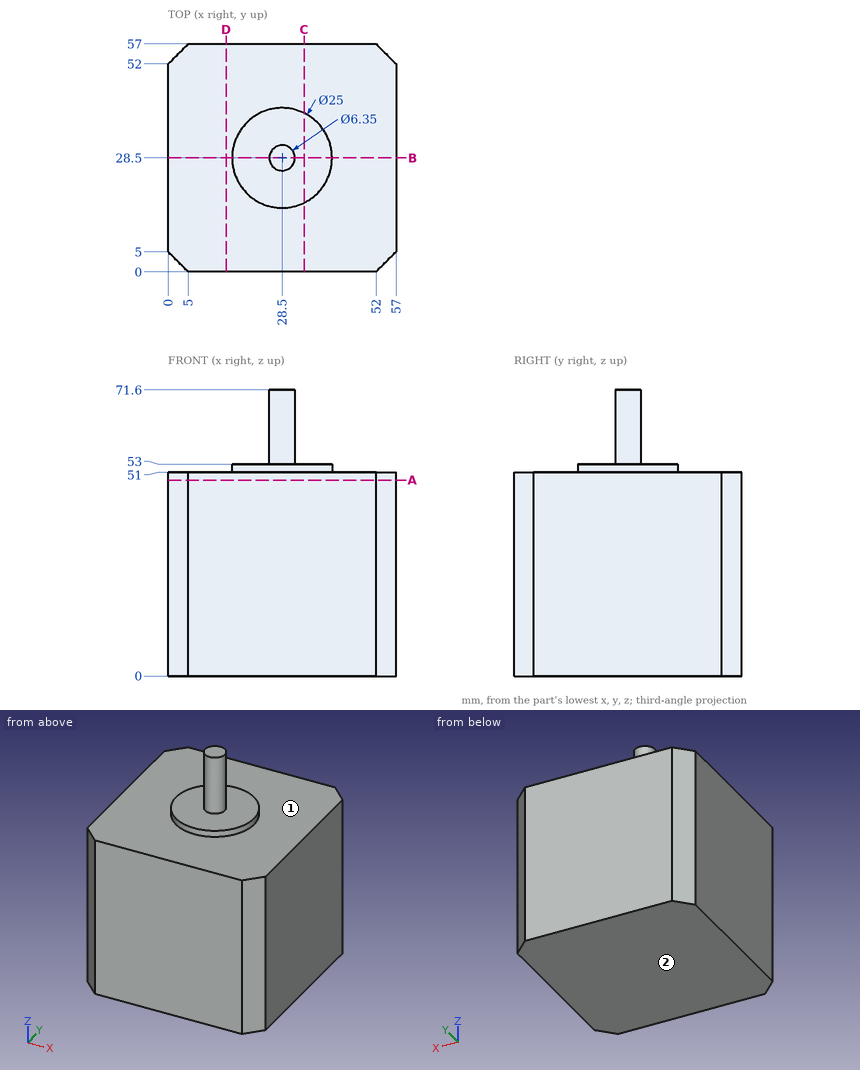
Input: dimensioned drawing with shaded views. Units: mm. Origin: part minimum x, y, z. A direction names the side the tool comes from. Coordinates: 2 decimals unless noted, no trailing zeros. Order: outer loops, then holes, each group sorted by start corner. A loop starts at its lowest first (then second) coordinate and runs counter-clockwise, first axis right, second up.
Item 1: Section query A-A (z = 49). Output: boundary loops of the cut face in (x, y), then the cut area to 3 significant figures.
Answer:
outline: (0, 5) - (5, 0) - (52, 0) - (57, 5) - (57, 52) - (52, 57) - (5, 57) - (0, 52) - close
area: 3,200 mm2
Item 2: Section query C-C (x = 34). Output: boundary loops of the cut face in (y, z).
Answer:
outline: (0, 0) - (57, 0) - (57, 51) - (39.72, 51) - (39.72, 53) - (17.28, 53) - (17.28, 51) - (0, 51) - close
Item 3: Section query B-B (y = 28.5). Output: boundary loops of the cut face in (x, z) (3 decimals).
Answer:
outline: (0, 0) - (57, 0) - (57, 51) - (41, 51) - (41, 53) - (31.675, 53) - (31.675, 71.6) - (25.325, 71.6) - (25.325, 53) - (16, 53) - (16, 51) - (0, 51) - close
Item 4: Section query D-D (x = 14.5). Output: boundary loops of the cut face in (y, z).
Answer:
outline: (0, 0) - (57, 0) - (57, 51) - (0, 51) - close
Item 5: Access query for the marked faces 1 and 2. Directions: +Z, -Z, +X, -X, +Y, -Y. A direction counts if a zero-diameter tool reaches every point of the face in a straight line with its end or side. Return the directions, or none.
Answer:
face 1: +Z
face 2: -Z, +X, -X, +Y, -Y
Item 6: Material intervals for line 1 along Z through (x, y) = (11.5, 20); line 2 along Z through (x, y) = (36.5, 36.5); line 3 along X through (y, z) = (4, 41), sorted ascending.
Answer:
line 1: z = 0 to 51
line 2: z = 0 to 53
line 3: x = 1 to 56
Item 7: Contact query for flat-ended pins moving along their axis: P1, Ø8, axis at y = 12, z = 17.5, coming from the -X side; P2, Ø4, axis at x = 30, y = 23.5, coming from the +Z side. Output: stop coordinate, or through.
Answer:
P1: stops at x = 0
P2: stops at z = 53
